Verification items for the finished model (mm, model axes). Coordinates: 2 decimals unless noted, no trailing zeros. Order: outer loops, then holes, each group sorted by start corner. A loop starts at its lowest first (then second) coordinate and runs counter-clockwise, first axis right, second up. Notation, with made-up numbers: M -20,-8 L -4,-8 A31 cw -4,26 Z; hole C -1.75,72 d9. An arc over 180 degrees is marked long. Return JSON: item names as keys, results as strings. Group by question number.
1. Gauge pin test, flat ends, axial feed: pin 1 (2 mm diameter, centred on x = 72, z = -63.5, fed in from +Y); pin 2 (1.5 mm diameter, centred on y = 6.5, z = -112, fed in from +X). Record the tip position at first contact, or that the pin passes through.
2. Section check B-B, the plane z = -108.6. Record the cut outline in (x, y).
3. Section check C-C, the plane x = 61. Record the cut outline in (y, z), plus the area to 3 significant figures.
4. Section check D-D, the plane y = 6.5. Record the cut outline in (x, z), plus the area to 3 significant figures.
5. Material ranges on line 1 along Y through (x, z) = (43, -75.5); line 2 along Z through (x, y) = (107.5, 2.25); line 3 along X through (y, z) = (5.5, -108.6), recorded low to high.
6. Section check A-A, the plane x = 108.6. Record the cut outline in (y, z).
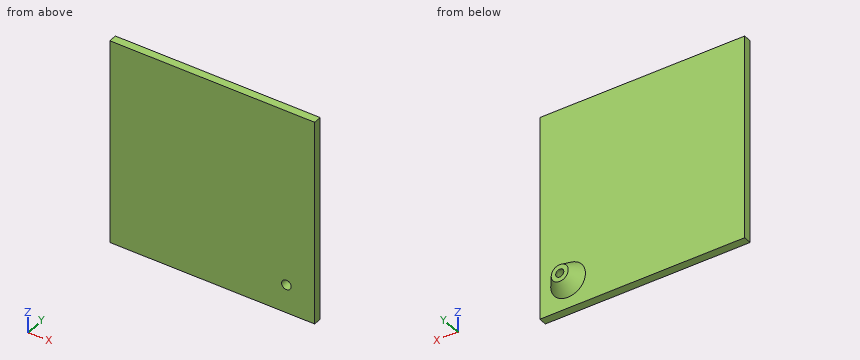
```python
from build123d import *

# Parameters (mm, degrees)
SKETCH1_W           = 126
SKETCH1_H           = 126
BOSS_EXTRUDE1_DEPTH = 5
SKETCH3_R           = 12.5
BOSS_EXTRUDE2_DEPTH = 7.5
SKETCH4_R           = 2.95
CUT_EXTRUDE1_DEPTH  = 11.5
SKETCH6_R           = 2.5
CUT_EXTRUDE2_DEPTH  = 179.628805068
CHAMFER1_SIZE       = 10
CHAMFER1_SIZE_2     = 7.26542528


with BuildPart() as part:
    # Sketch1 → Boss-Extrude1 (new body)
    with BuildSketch(Plane(origin=(0, 0, 0), x_dir=(1, 0, 0), z_dir=(0, 1, 0))):
        with Locations((63, 63)):
            Rectangle(SKETCH1_W, SKETCH1_H)
    extrude(amount=BOSS_EXTRUDE1_DEPTH)

    # Sketch3 → Boss-Extrude2 (add)
    with BuildSketch(Plane(origin=(0, 5, 0), x_dir=(1, 0, 0), z_dir=(0, 1, 0))):
        with Locations(Location((108.6, 108.6, 0), (0, 0, 90))):
            Circle(SKETCH3_R)
    extrude(amount=BOSS_EXTRUDE2_DEPTH)

    # Sketch4 → Cut-Extrude1 (cut)
    with BuildSketch(Plane.XZ):
        with Locations(Location((108.6, -108.6, 0), (0, 0, 270))):
            Circle(SKETCH4_R)
    extrude(amount=-CUT_EXTRUDE1_DEPTH, mode=Mode.SUBTRACT)

    # Sketch6 → Cut-Extrude2 (cut, through all)
    with BuildSketch(Plane(origin=(0, 12.5, 0), x_dir=(1, 0, 0), z_dir=(0, 1, 0))):
        with Locations(Location((108.6, 108.6, 0), (0, 0, 270))):
            Circle(SKETCH6_R)
    extrude(amount=-CUT_EXTRUDE2_DEPTH, mode=Mode.SUBTRACT)

    # Chamfer1
    # the kernel refuses this chamfer: 10, 7.26542528 mm, written as the material it takes off along each edge
    with BuildSketch(Plane(origin=(108.6, 12.5, -108.6), x_dir=(0, 0, -1), z_dir=(1, 0, 0))) as chamfer1_piece_1_section:
        Polygon((12.5, -CHAMFER1_SIZE), (12.5 - CHAMFER1_SIZE_2, 0), (12.5, 0), align=None)
    chamfer1_piece_1 = revolve(axis=Axis((108.6, 12.5, -108.6), (0, 1, 0)), mode=Mode.PRIVATE)
    chamfer1_piece_1 = split(chamfer1_piece_1, bisect_by=Plane(origin=(108.6, 5, -100.650989912), z_dir=(0, 1, 0)), keep=Keep.TOP, mode=Mode.PRIVATE)
    add(chamfer1_piece_1, mode=Mode.SUBTRACT)


solid = part.part
```
Answers follow:
{
 "1": {"pin 1": "y = 5", "pin 2": "x = 118.21"},
 "2": {"outline": "M 0,0 L 105.65,0 L 105.65,11.5 L 106.1,11.5 L 106.1,12.5 L 103.37,12.5 L 97.92,5 L 0,5 Z; M 111.1,11.5 L 111.55,11.5 L 111.55,0 L 126,0 L 126,5 L 119.28,5 L 113.83,12.5 L 111.1,12.5 Z"},
 "3": {"outline": "M 0,-126 L 5,-126 L 5,0 L 0,0 Z", "area": "630 mm^2"},
 "4": {"outline": "C 108.6,-108.6 d19.19; hole C 108.6,-108.6 d5.9", "area": "262 mm^2"},
 "5": {"line 1": "0 to 5", "line 2": "-126 to -111.34, -105.86 to 0", "line 3": "98.28 to 105.65, 111.55 to 118.92"},
 "6": {"outline": "M 0,-126 L 5,-126 L 5,-119.28 L 12.5,-113.83 L 12.5,-111.1 L 11.5,-111.1 L 11.5,-111.55 L 0,-111.55 Z; M 0,-105.65 L 11.5,-105.65 L 11.5,-106.1 L 12.5,-106.1 L 12.5,-103.37 L 5,-97.92 L 5,0 L 0,0 Z"}
}
